from build123d import *

# Parameters (mm, degrees)
SKETCH1_R             = 13
BOSS_EXTRUDE1_DEPTH   = 25
BOSS_EXTRUDE2_DEPTH   = 7.5
BOSS_EXTRUDE2_2_DEPTH = 7.5
BOSS_EXTRUDE3_DEPTH   = 15
SKETCH5_R             = 3
CUT_EXTRUDE1_DEPTH    = 40.389084782
SKETCH6_R             = 4.45
CUT_EXTRUDE2_DEPTH    = 3
SKETCH7_R             = 4
CUT_EXTRUDE3_DEPTH    = 7.5
SKETCH8_W             = 50
SKETCH8_H             = 50
CUT_EXTRUDE4_DEPTH    = 37.058979464


with BuildPart() as part:
    # Sketch1 → Boss-Extrude1 (new body)
    with BuildSketch(Plane.XY):
        Circle(SKETCH1_R)
    extrude(amount=-BOSS_EXTRUDE1_DEPTH)

    # Sketch2 → Cut-Revolve1 (revolve, cut)
    with BuildSketch(Plane(origin=(0, 0, 0), x_dir=(0, 0, -1), z_dir=(1, 0, 0)), mode=Mode.PRIVATE) as cut_revolve1_sk:
        Polygon((0, 0), (0, 7.6), (11.5, 9.5), (14, 10.6), (25, 11), (25, 0), align=None)
    revolve(cut_revolve1_sk.sketch.rotate(Axis((0, 0, -25), (0, 0, 1)), 90), axis=Axis((0, 0, -25), (0, 0, 1)), mode=Mode.SUBTRACT)



with BuildPart() as body_2:
    # Sketch3 → Boss-Extrude2 (new, symmetric)
    with BuildSketch(Plane(origin=(0, 0, 0), x_dir=(1, 0, 0), z_dir=(0, 1, 0))):
        with BuildLine():
            Line((-13, 25), (-13, 10))
            Line((-13, 10), (-15, 10))
            ThreePointArc((-15, 10), (-22.5, 17.5), (-15, 25))
            Line((-15, 25), (-13, 25))
        make_face()
    extrude(amount=BOSS_EXTRUDE2_DEPTH, both=True)


with BuildPart() as body_3:
    # Sketch3 → Boss-Extrude2 2 (new, symmetric)
    with BuildSketch(Plane(origin=(0, 0, 0), x_dir=(1, 0, 0), z_dir=(0, 1, 0))):
        with BuildLine():
            Line((13, 25), (15, 25))
            ThreePointArc((15, 25), (22.5, 17.5), (15, 10))
            Line((15, 10), (13, 10))
            Line((13, 10), (13, 25))
        make_face()
    extrude(amount=BOSS_EXTRUDE2_2_DEPTH, both=True)


with BuildPart() as part_1:
    add(part.part)

    add(body_2.part)  # Boss-Extrude3 merges body 2

    add(body_3.part)  # Boss-Extrude3 merges body 3
    # Sketch4 → Boss-Extrude3 (add)
    with BuildSketch(Plane(origin=(0, 0, -25), x_dir=(-1, 0, 0), z_dir=(0, 0, -1))):
        with BuildLine():
            Line((-13, 7.5), (-13, -7.5))
            Line((-13, -7.5), (-8.04673847, -7.5))
            ThreePointArc((-8.04673847, -7.5), (-11, 0), (-8.04673847, 7.5))
            Line((-8.04673847, 7.5), (-13, 7.5))
        make_face()
        with BuildLine():
            Line((13, 7.5), (13, -7.5))
            Line((13, -7.5), (8.04673847, -7.5))
            ThreePointArc((8.04673847, -7.5), (11, 0), (8.04673847, 7.5))
            Line((8.04673847, 7.5), (13, 7.5))
        make_face()
    extrude(amount=-BOSS_EXTRUDE3_DEPTH)

    # Sketch5 → Cut-Extrude1 (cut, through all)
    with BuildSketch(Plane(origin=(0, 7.5, 0), x_dir=(1, 0, 0), z_dir=(0, 1, 0))):
        with Locations(Location((16.9, 17.5, 0), (0, 0, 270))):
            Circle(SKETCH5_R)
        with Locations(Location((-16.9, 17.5, 0), (0, 0, 270))):
            Circle(SKETCH5_R)
    extrude(amount=-CUT_EXTRUDE1_DEPTH, mode=Mode.SUBTRACT)

    # Sketch6 → Cut-Extrude2 (cut)
    with BuildSketch(Plane(origin=(0, 7.5, 0), x_dir=(1, 0, 0), z_dir=(0, 1, 0))):
        with Locations(Location((-16.9, 17.5, 0), (0, 0, 270))):
            Circle(SKETCH6_R)
        with Locations(Location((16.9, 17.5, 0), (0, 0, 270))):
            Circle(SKETCH6_R)
    extrude(amount=-CUT_EXTRUDE2_DEPTH, mode=Mode.SUBTRACT)

    # Sketch7 → Cut-Extrude3 (cut)
    with BuildSketch(Plane.XZ.offset(7.5)):
        with Locations(Location((-16.9, -17.5, 0), (0, 0, 270))):
            Circle(SKETCH7_R)
        with Locations(Location((16.9, -17.5, 0), (0, 0, 270))):
            Circle(SKETCH7_R)
    extrude(amount=-CUT_EXTRUDE3_DEPTH, mode=Mode.SUBTRACT)

    # Sketch8 → Cut-Extrude4 (cut, through all)
    with BuildSketch(Plane(origin=(0, 0, 0), x_dir=(1, 0, 0), z_dir=(0, 1, 0))):
        with Locations((0, 14.017641389)):
            Rectangle(SKETCH8_W, SKETCH8_H)
    extrude(amount=CUT_EXTRUDE4_DEPTH, mode=Mode.SUBTRACT)


solid = part_1.part
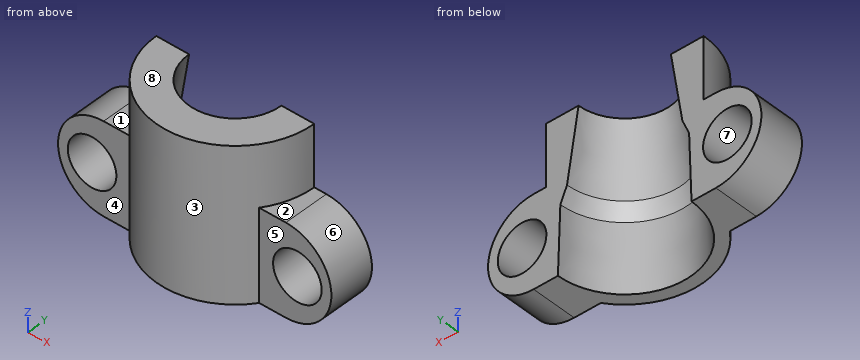
Design review of the part built by this model. Coordinates are the model's own, in mm. Face numbers are marked on the shaded views. A direction names the side the tool comes from. Coordinates: 2 decimals unless noted, no trailing zeros. Loops run counter-clockwise (first coordinate to the right, second up) from the corner with the lowest first, then second, coordinate; pieces in that order, holes last. Notation, with made-up numbers: (8.25, -2) - (21.25, -2) arc R13 cw to (21.25, 8) - close; hole circle Ø7 at (-5.75, 44.5). An arc over 180 degrees is marked (long way). Use CSV: the item, a comma, the result in double quotes. Start each with the question number.
1. Add section C-C on y = -1. Count the separate pieces of the cut face and the enclosed holes in it, plus the area to 3 significant figures.
2. Add section A-A on z = -19.5. Give the boundary of the cut face in (x, y).
3. For the marked faces 1, 2, 3, 4 and 5, list the 3-axis set-ups (+Z, -Z, +X, -X, +Y, -Y) from which the entire face can be reached by the end or side of a thin tool; tool diameter is ignored.
4. Clearance check with flat-ended pins moving along their axes: pin 1 (2 mm diameter, centred on x = 16.5, y = -4.5, fed in from -Z); pin 2 (3 mm diameter, centred on y = -6, z = -2.5, fed in from +X); pin 3 (13 mm diameter, centred on x = -14.5, z = -19, fed in from -Y). State where each tip first meets the part, or that it passes through.
5. Add section D-D on x = 0. Give the boundary of the cut face in (y, z), plus the area to 4 significant figures.
6. To check wall thickness, follow probe 1 along X at (y, z) = (-3.5, -17.5); probe 2 along X at (y, z) = (-1.5, -17.5); probe 3 along Y at (x, z) = (-13, -10.25). State the ranges of each line that lie inside material, in increasing order.
7. Add section B-B on x = -16. Give the boundary of the cut face in (y, z).
8. Mouldability with a two-part tool opening along X and no side actions: class the marked faces 6, 7 and 8 as released by +X, released by -X, zero draft, split by the parting line, or undercut.
Resolved:
1,separate pieces,"2"
1,enclosed holes,"2"
1,area,"304 mm2"
2,outline,"(-22.23, -7.5) - (-20.36, -7.5) - (-20.36, 0) - (-22.23, 0) - close; (-13.44, -7.5) - (-10.62, -7.5) arc R13 ccw to (10.62, -7.5) - (13.44, -7.5) - (13.44, 0) - (10.8, 0) arc R10.8 cw to (-10.8, 0) - (-13.44, 0) - close; (20.36, -7.5) - (22.23, -7.5) - (22.23, 0) - (20.36, 0) - close"
3,face 1,"+Z, -X, -Y"
3,face 2,"+Z, +X, -Y"
3,face 3,"+Z, -Y"
3,face 4,"+Z, -Z, -X, -Y"
3,face 5,"+Z, -Z, +X, -Y"
4,pin 1,"z = -24.98"
4,pin 2,"x = 12.2"
4,pin 3,"y = -10.25"
5,outline,"(-13, -25) - (-11, -25) - (-10.6, -14) - (-9.5, -11.5) - (-7.6, 0) - (-13, 0) - close"
5,area,"82.75 mm2"
6,probe 1,"-22.5 to -20.9, -12.9 to -10.14, 10.14 to 12.9, 20.9 to 22.5"
6,probe 2,"-22.5 to -20.9, -12.9 to -10.62, 10.62 to 12.9, 20.9 to 22.5"
6,probe 3,"-7.5 to 0"
7,outline,"(-7.5, -24.93) - (0, -24.93) - (0, -21.4) - (-7.5, -21.4) - close; (-7.5, -13.6) - (0, -13.6) - (0, -10.07) - (-7.5, -10.07) - close"
8,face 6,"released by +X"
8,face 7,"undercut"
8,face 8,"zero draft"
